```python
from build123d import *

# Parameters (mm, degrees)
SKETCH1_W           = 80
SKETCH1_H           = 90
SKETCH1_R           = 1.75
BOSS_EXTRUDE1_DEPTH = 4
SKETCH2_W           = 80
SKETCH2_H           = 90
BOSS_EXTRUDE2_DEPTH = 50
SKETCH3_W           = 5
SKETCH3_H           = 15
CUT_EXTRUDE1_DEPTH  = 40
SKETCH6_W           = 10
SKETCH6_H           = 50
SKETCH6_W_2         = 7.5
CUT_EXTRUDE5_DEPTH  = 159.164471358
SKETCH8_W           = 10
SKETCH8_H           = 49
CUT_EXTRUDE6_DEPTH  = 159.164471358


with BuildPart() as part:
    # Sketch1 → Boss-Extrude1 (new body)
    with BuildSketch(Plane(origin=(0, 0, 0), x_dir=(1, 0, 0), z_dir=(0, 1, 0))):
        Polygon((0, 0), (90, 0), (90, 45), (110, 45), (110, 55), (90, 55), (90, 100), (0, 100), (0, 55), (-20, 55), (-20, 45), (0, 45), align=None)
        with Locations((45, 50)):
            Rectangle(SKETCH1_W, SKETCH1_H, mode=Mode.SUBTRACT)
        with Locations(Location((-10, 50, 0), (0, 0, 270))):
            Circle(SKETCH1_R, mode=Mode.SUBTRACT)
        with Locations(Location((100, 50, 0), (0, 0, 270))):
            Circle(SKETCH1_R, mode=Mode.SUBTRACT)
    extrude(amount=BOSS_EXTRUDE1_DEPTH)

    # Sketch2 → Boss-Extrude2 (add)
    with BuildSketch(Plane(origin=(0, 4, 0), x_dir=(1, 0, 0), z_dir=(0, 1, 0))):
        Polygon((0, 45), (0, 0), (90, 0), (90, 45), (90, 55), (90, 100), (0, 100), (0, 55), align=None)
        with Locations((45, 50)):
            Rectangle(SKETCH2_W, SKETCH2_H, mode=Mode.SUBTRACT)
    extrude(amount=BOSS_EXTRUDE2_DEPTH)

    # Sketch3 → Cut-Extrude1 (cut)
    with BuildSketch(Plane(origin=(0, 54, 0), x_dir=(1, 0, 0), z_dir=(0, 1, 0))):
        with Locations((87.5, 50)):
            Rectangle(SKETCH3_W, SKETCH3_H)
        with Locations((2.5, 50)):
            Rectangle(SKETCH3_W, SKETCH3_H)
    extrude(amount=-CUT_EXTRUDE1_DEPTH, mode=Mode.SUBTRACT)

    # Sketch6 → Cut-Extrude5 (cut, through all)
    with BuildSketch(Plane(origin=(0, 0, -100), x_dir=(-1, 0, 0), z_dir=(0, 0, -1))):
        with Locations((-80, 29)):
            Rectangle(SKETCH6_W, SKETCH6_H)
        with Locations((-65, 29)):
            Rectangle(SKETCH6_W, SKETCH6_H)
        with Locations((-51.25, 29)):
            Rectangle(SKETCH6_W_2, SKETCH6_H)
        with Locations((-38.75, 29)):
            Rectangle(SKETCH6_W_2, SKETCH6_H)
        with Locations((-25, 29)):
            Rectangle(SKETCH6_W, SKETCH6_H)
        with Locations((-10, 29)):
            Rectangle(SKETCH6_W, SKETCH6_H)
    extrude(amount=-CUT_EXTRUDE5_DEPTH, mode=Mode.SUBTRACT)

    # Sketch8 → Cut-Extrude6 (cut, through all)
    with BuildSketch(Plane(origin=(90, 0, 0), x_dir=(0, 0, -1), z_dir=(1, 0, 0))):
        with Locations((10, 29.5)):
            Rectangle(SKETCH8_W, SKETCH8_H)
        with Locations((25, 29.5)):
            Rectangle(SKETCH8_W, SKETCH8_H)
        Polygon((42.5, 54), (35, 54), (35, 5), (42.5, 5), (42.5, 14), align=None)
        Polygon((57.5, 14), (57.5, 5), (65, 5), (65, 54), (57.5, 54), align=None)
        with Locations((75, 29.5)):
            Rectangle(SKETCH8_W, SKETCH8_H)
        with Locations((90, 29.5)):
            Rectangle(SKETCH8_W, SKETCH8_H)
    extrude(amount=-CUT_EXTRUDE6_DEPTH, mode=Mode.SUBTRACT)


solid = part.part
```
Here's how the part is built. I have some questions about the finished solid (model axes, mm). A direction names the side the tool comes from. Round coordinates to 2 decimals unless told otherwise and drop trailing zeros. Loops run counter-clockwise (first coordinate to the right, second up) from the corner with the lowest first, then second, coordinate; pieces in that order, holes last. Notation, with made-up numbers: (-26, 55) -> (-15, 55) arc R14 cw to (-15, 82) -> close; hole circle Ø7 at (-1, 66). An arc over 180 degrees is marked (long way). Answer as CSV lines item,"result". Start each with the question number.
1. Imagine slicing it at C-C on z = -50. Write out the boundary of the cut face in (x, y).
2. I'm going to push flat-ended pins straight in: P1, Ø1.5, axis at y = 35, z = -98.5, coming from the +X side; P2, Ø12, axis at y = 24, z = -46, coming from the -X side; P3, Ø10, axis at x = 84, y = 33.5, coming from the +Z side; P4, Ø4.5, axis at x = -9, y = 2.5, coming from the +Z side. Where does each tip first touch, or does it pass through?
3. Imagine slicing it at D-D on x = 88. Write out the boundary of the cut face in (y, z).
4. I need wall thicknesses on probe 1 along X at (y, z) = (1, -50); probe 2 along X at (y, z) = (21, -67.5); probe 3 along Z at (x, y) = (31.5, 11). Which ranges of each line are inside material? Lowest first, please. Write a range as from..to.
5. If we mould it in two halves opening along X, with no side actions, what happens to faces 4 (the face through (87, 54, -98)), 5 (the face through (80, 4, -98))? For each: pulls with the +X half, pulls with the -X half, needs draft (parallel to the pull), parting line crosses it, or undercut.
6. For faces 1 (the face through (35, 29, -3)), 2 (the face through (57, 54, -3)), 3 (the face through (88, 5, -61)), which set-ups out of +Z, -Z, +X, -X, +Y, -Y let a thin tool reach every point of the face, with its end or its side?
7. Imagine slicing it at A-A on z = -13.5. Write out the boundary of the cut face in (x, y).
8. Imagine slicing it at B-B on x = 46. Write out the boundary of the cut face in (y, z).
Solution:
1,outline,"(-20, 0) -> (-11.75, 0) -> (-11.75, 4) -> (-20, 4) -> close; (-8.25, 0) -> (5, 0) -> (5, 14) -> (0, 14) -> (0, 4) -> (-8.25, 4) -> close; (85, 0) -> (98.25, 0) -> (98.25, 4) -> (90, 4) -> (90, 14) -> (85, 14) -> close; (101.75, 0) -> (110, 0) -> (110, 4) -> (101.75, 4) -> close"
2,P1,"x = 90"
2,P2,"through"
2,P3,"z = 0"
2,P4,"z = -45"
3,outline,"(0, -100) -> (54, -100) -> (54, -95) -> (5, -95) -> (5, -85) -> (54, -85) -> (54, -80) -> (5, -80) -> (5, -70) -> (54, -70) -> (54, -65) -> (5, -65) -> (5, -57.5) -> (14, -57.5) -> (14, -42.5) -> (5, -42.5) -> (5, -35) -> (54, -35) -> (54, -30) -> (5, -30) -> (5, -20) -> (54, -20) -> (54, -15) -> (5, -15) -> (5, -5) -> (54, -5) -> (54, 0) -> (0, 0) -> close"
4,probe 1,"-20..-11.75, -8.25..5, 85..98.25, 101.75..110"
4,probe 2,"0..5, 85..90"
4,probe 3,"-100..-95, -5..0"
5,face 4,"needs draft"
5,face 5,"undercut"
6,face 1,"+Z, -Z, +Y"
6,face 2,"+Z, -Z, +X, -X, +Y"
6,face 3,"+X, -X, +Y"
7,outline,"(0, 0) -> (5, 0) -> (5, 5) -> (0, 5) -> close; (85, 0) -> (90, 0) -> (90, 5) -> (85, 5) -> close"
8,outline,"(0, -100) -> (54, -100) -> (54, -95) -> (0, -95) -> close; (0, -5) -> (54, -5) -> (54, 0) -> (0, 0) -> close"
